Here's the drawing with two shaded views (mm, measured from the low corner). I have some questions. Round coordinates to 2 decimals unless told otherwise and drop trailing zeros. Order: outer loops, then holes, each group sorted by start corner. A loop starts at its lowest first (then second) coordinate and runs counter-clockwise, first axis right, second up. Notation, with made-up numbers: M -40,50 L 14,50 A22 ccw 14,66 Z; hole C 30.5,-7.5 d8. An arc over 180 degrees is marked long. One line per question, with ' | ' between items.
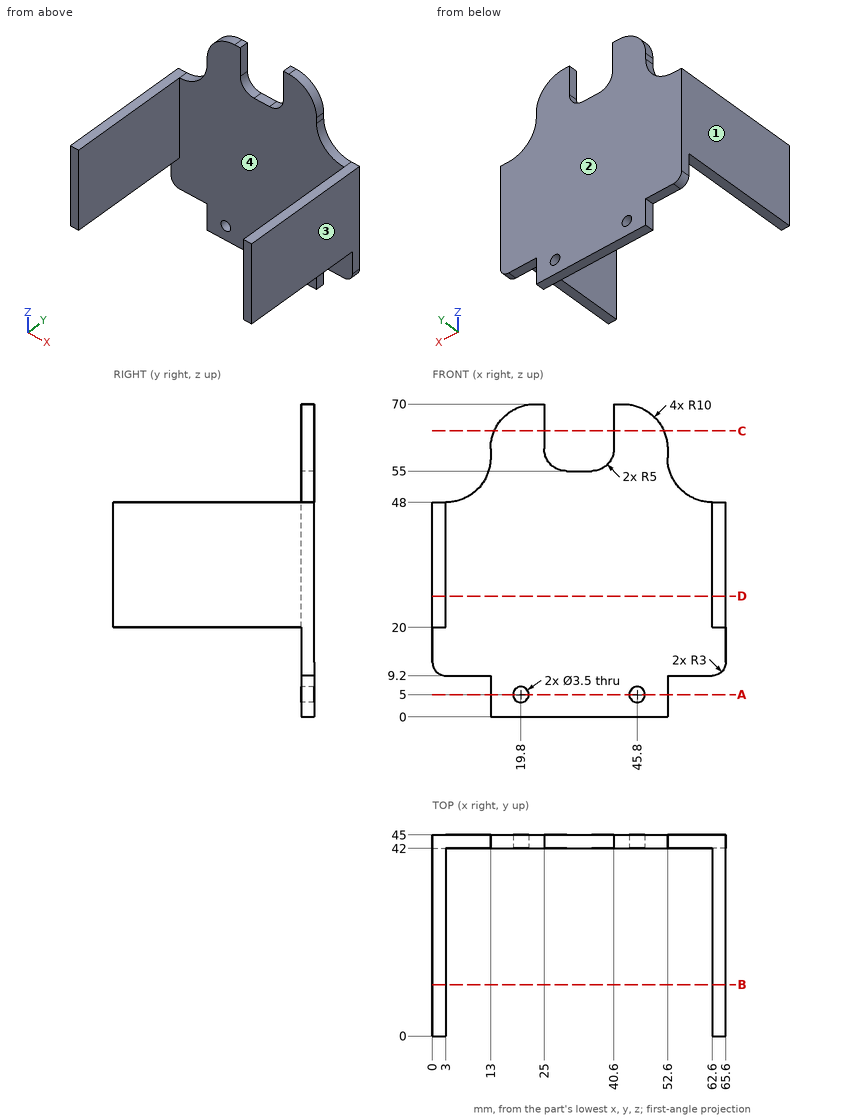
(1) If we section it at C-C on z = 64: Please give me the cut outline in (x, y).
Final values:
outline: M 13.83,42 L 25,42 L 25,45 L 13.83,45 Z; M 40.6,42 L 51.77,42 L 51.77,45 L 40.6,45 Z
(2) If we section it at A-A on z = 5: Please give me the cut outline in (x, y).
Final values:
outline: M 13,42 L 18.05,42 L 18.05,45 L 13,45 Z; M 21.55,42 L 44.05,42 L 44.05,45 L 21.55,45 Z; M 47.55,42 L 52.6,42 L 52.6,45 L 47.55,45 Z
(3) Please list where these lines run through material, in increasing order: probe 1 along X at (y, z) = (44.2, 5); probe 2 along X at (y, z) = (3.5, 37); probe 3 along Y at (x, z) = (43.5, 60.5). Write a range as [from, to].
Final values:
probe 1: [13, 18.05], [21.55, 44.05], [47.55, 52.6] | probe 2: [0, 3], [62.6, 65.6] | probe 3: [42, 45]
(4) If we section it at D-D on z = 27: Please give me the cut outline in (x, y), plus the area to 3 significant figures.
Final values:
outline: M 0,0 L 3,0 L 3,42 L 62.6,42 L 62.6,0 L 65.6,0 L 65.6,45 L 0,45 Z | area: 449 mm^2
(5) Thinking about a two-plate mould opening in X: for the marked faces 1, 2, 3 and 4, which applies, released by +X, released by -X, zero draft, split by the parting line, or undercut?
Final values:
face 1: released by -X | face 2: zero draft | face 3: released by +X | face 4: undercut
(6) Will these pins go through, and if not, where does the flat tip stop? pin 1 Ø3.5 at (x, y) = (7.5, 43) entering from -Z; pin 2 Ø1.5 at (y, z) = (44, 65.5) entering from -X; pin 3 Ø1.5 at (x, y) = (33, 43) entering from +Z; pin 4 Ø22.5 at (y, z) = (12.5, 40.5) entering from -X.
Final values:
pin 1: z = 9.2 | pin 2: x = 14.2 | pin 3: z = 55 | pin 4: x = 0
(7) If we section it at B-B on y = 11.5: Please give me the cut outline in (x, z).
Final values:
outline: M 0,20 L 3,20 L 3,48 L 0,48 Z; M 62.6,20 L 65.6,20 L 65.6,48 L 62.6,48 Z
